Here's how the part is built. I have some questions about the finished solid (model axes, mm). Round coordinates to 2 decimals unless told otherwise and drop trailing zeros. Loops run counter-clockwise (first coordinate to the right, second up) from the corner with the lowest first, then second, coordinate; pieces in that order, holes last. Notation, with made-up numbers: (70.25, -1) - (94.25, -1) arc R22 cw to (94.25, 38) - close; hole circle Ø7 at (35.5, 7.25). An arc over 180 degrees is marked (long way). Answer as a JSON object with one key per item and string values. Group by question number.
1) I want a section at A-A, the plane z = -6. Please give me the cut outline in (x, y) (3 decimals).
2) I want a section at C-C, the plane y = 1. Please give me the cut outline in (x, z) (1 decimal).
3) If I drill on line 1 along Z through (x, y) = (93, 1.95); line 2 along Z through (x, y) = (-64, 1.35); line 3 along Z through (x, y) = (29, 2.9), over which ranges is the centre line in solid material (lowest first)? Write a range as [from, to].
4) Will these pins go through, and if not, where does the flat tip stop? P1, Ø1, axis at y = 2, z = -11.5, coming from the +X side; P2, Ø2.5, axis at x = 107.79, z = 17.08, coming from the +Y side.
5) I want a section at D-D, the plane x = 2.5. Please give me the cut outline in (y, z) (3 decimals).
6) I want a section at B-B, the plane x = 92.5. Please give me the cut outline in (y, z) (3 decimals).
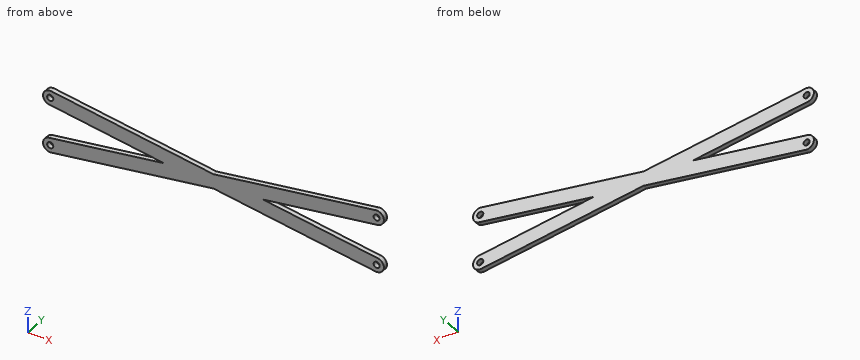
from build123d import *

# Parameters (mm, degrees)
BOSS_EXTRUDE1_DEPTH = 3.175
SKETCH2_R           = 2.032
CUT_EXTRUDE1_DEPTH  = 115.695104393


with BuildPart() as part:
    # Sketch1 → Boss-Extrude1 (new body)
    with BuildSketch(Plane(origin=(0, 0, 0), x_dir=(1, 0, 0), z_dir=(0, 1, 0))):
        with BuildLine():
            Line((-108.172056186, -12.373235341), (-32.483719252, -1.209763817))
            Line((-32.483719252, -1.209763817), (-108.172056172, 9.953707462))
            ThreePointArc((-108.172056172, 9.953707462), (-112.188668788, 15.360151236), (-106.782225129, 19.376764008))
            Line((-106.782225129, 19.376764008), (0.155358302, 3.604259421))
            Line((0.155358302, 3.604259421), (107.092941684, 19.376764345))
            ThreePointArc((107.092941684, 19.376764345), (112.499387579, 15.360153144), (108.482775156, 9.953708157))
            Line((108.482775156, 9.953708157), (32.794435872, -1.209763714))
            Line((32.794435872, -1.209763714), (108.482775141, -12.373235339))
            ThreePointArc((108.482775141, -12.373235339), (112.499387585, -17.779680288), (107.092941749, -21.796291538))
            Line((107.092941749, -21.796291538), (0.155358318, -6.023786952))
            Line((0.155358318, -6.023786952), (-106.782225064, -21.796291875))
            ThreePointArc((-106.782225064, -21.796291875), (-112.188668782, -17.779679153), (-108.172056186, -12.373235341))
        make_face()
    extrude(amount=BOSS_EXTRUDE1_DEPTH)

    # Sketch2 → Cut-Extrude1 (cut, through all)
    with BuildSketch(Plane(origin=(0, 3.175, 0), x_dir=(1, 0, 0), z_dir=(0, 1, 0))):
        with Locations(Location((-107.477140515, 14.665235715, 0), (0, 0, 270))):
            Circle(SKETCH2_R)
        with Locations(Location((-107.477140515, -17.084763592, 0), (0, 0, 270))):
            Circle(SKETCH2_R)
        with Locations(Location((107.787859485, 14.665236408, 0), (0, 0, 270))):
            Circle(SKETCH2_R)
        with Locations(Location((107.787859485, -17.084763592, 0), (0, 0, 270))):
            Circle(SKETCH2_R)
    extrude(amount=-CUT_EXTRUDE1_DEPTH, mode=Mode.SUBTRACT)


solid = part.part
Outcome:
{
 "1": {"outline": "(-81.366, 0) - (-16.088, 0) - (-16.088, 3.175) - (-81.366, 3.175) - close; (16.398, 0) - (81.677, 0) - (81.677, 3.175) - (16.398, 3.175) - close"},
 "2": {"outline": "(-108.2, -10) arc R4.8 ccw to (-106.8, -19.4) - (0.2, -3.6) - (107.1, -19.4) arc R4.8 ccw to (108.5, -10) - (32.8, 1.2) - (108.5, 12.4) arc R4.8 ccw to (107.1, 21.8) - (0.2, 6) - (-106.8, 21.8) arc R4.8 ccw to (-108.2, 12.4) - (-32.5, 1.2) - close; hole circle Ø4.1 at (-107.5, -14.7); hole circle Ø4.1 at (-107.5, 17.1); hole circle Ø4.1 at (107.8, -14.7); hole circle Ø4.1 at (107.8, 17.1)"},
 "3": {"line 1": "[-17.3, -7.67], [10.09, 19.72]", "line 2": "[-13.07, -3.44], [5.86, 15.49]", "line 3": "[-7.86, 10.28]"},
 "4": {"P1": "x = 111.73", "P2": "through"},
 "5": {"outline": "(0, -3.95) - (3.175, -3.95) - (3.175, 6.37) - (0, 6.37) - close"},
 "6": {"outline": "(0, -17.224) - (3.175, -17.224) - (3.175, -7.596) - (0, -7.596) - close; (0, 10.016) - (3.175, 10.016) - (3.175, 19.644) - (0, 19.644) - close"}
}
